Can you work these out from the model? Positions are in its coordinate system, mm. A direction names the side the tool comes from. Give positions to 0.01 mm unless a question says otherwise; leave off trailing zeros. Loops run counter-clockwise (first coordinate to the right, second up) from the corner with the lowest first, then second, coordinate; pieces in that order, holes last.
from build123d import *

# Parameters (mm, degrees)
SKETCH_1_R           = 6
EXTRUDE_1_DEPTH      = 2
SKETCH_2_R           = 3.5
EXTRUDE_2_DEPTH      = 12.5
EXTRUDE_START        = -2.5
EXTRUDE_3_DEPTH      = 2.5
EXTRUDE_4_DEPTH      = 0.5
EXTRUDE_4_DEPTH_BACK = 0.5
SKETCH_5_R           = 3
EXTRUDE_5_DEPTH      = 0.5
SKETCH_6_R           = 2
EXTRUDE_6_DEPTH      = 16
SKETCH_8_W           = 1
SKETCH_8_H           = 6
CUT_EXTRUDE_1_DEPTH  = 6
CUT_EXTRUDE_2_DEPTH  = 24.092206478
FILLET_1_R           = 0.2
CHAMFER_1_SIZE       = 0.5


with BuildPart() as part:
    # 草图1 → 凸台-拉伸1 (new body)
    with BuildSketch(Plane(origin=(0, 0, 0), x_dir=(1, 0, 0), z_dir=(0, 1, 0))):
        with Locations(Location((0, 0, 0), (0, 0, 270))):
            Circle(SKETCH_1_R)
    extrude(amount=EXTRUDE_1_DEPTH)

    # 草图2 → 凸台-拉伸2 (add)
    with BuildSketch(Plane(origin=(0, 2, 0), x_dir=(1, 0, 0), z_dir=(0, 1, 0))):
        with Locations(Location((0, 0, 0), (0, 0, 270))):
            Circle(SKETCH_2_R)
    extrude(amount=EXTRUDE_2_DEPTH)

    # 草图3 → 凸台-拉伸3 (add)
    with BuildSketch(Plane(origin=(0, 14.5, 0), x_dir=(1, 0, 0), z_dir=(0, 1, 0)).offset(EXTRUDE_START)):
        with BuildLine():
            Line((-12.125, 2.997394702), (-0.145833333, 3.496960486))
            ThreePointArc((-0.145833333, 3.496960486), (3.5, 0), (-0.145833333, -3.496960486))
            Line((-0.145833333, -3.496960486), (-12.125, -2.997394702))
            ThreePointArc((-12.125, -2.997394702), (-15, 0), (-12.125, 2.997394702))
        make_face()
    extrude(amount=EXTRUDE_3_DEPTH)

    # 草图4 → 凸台-拉伸4 (add, two sides: drawn at the far end of the back side and taken through both)
    with BuildSketch(Plane.XY.offset(-EXTRUDE_4_DEPTH_BACK)):
        Polygon((-14.2, 12), (-3.2, 8), (-0.2, 6.909090909), (-0.2, 12), (-3.2, 12), align=None)
    extrude(amount=EXTRUDE_4_DEPTH + EXTRUDE_4_DEPTH_BACK)

    # 草图5 → 凸台-拉伸5 (add)
    with BuildSketch(Plane(origin=(0, 14.5, 0), x_dir=(1, 0, 0), z_dir=(0, 1, 0))):
        with Locations(Location((-12, 0, 0), (0, 0, 270))):
            Circle(SKETCH_5_R)
    extrude(amount=EXTRUDE_5_DEPTH)

    # 草图6 → 凸台-拉伸6 (add)
    with BuildSketch(Plane(origin=(0, 15, 0), x_dir=(1, 0, 0), z_dir=(0, 1, 0))):
        with Locations(Location((-12, 0, 0), (0, 0, 270))):
            Circle(SKETCH_6_R)
    extrude(amount=EXTRUDE_6_DEPTH)

    # 草图7 → 旋转1 (revolve)
    with BuildSketch(Plane.XY, mode=Mode.PRIVATE) as revolve_1_sk:
        Polygon((-12, 31), (-14, 31), (-14.1, 30), (-12, 30), align=None)
    revolve(revolve_1_sk.sketch.rotate(Axis((-12, 30, 0), (0, 1, 0)), 90), axis=Axis((-12, 30, 0), (0, 1, 0)))

    # 草图8 → 切除-拉伸1 (cut)
    with BuildSketch(Plane(origin=(0, 31, 0), x_dir=(1, 0, 0), z_dir=(0, 1, 0))):
        with Locations((-12, 0)):
            Rectangle(SKETCH_8_W, SKETCH_8_H)
    extrude(amount=-CUT_EXTRUDE_1_DEPTH, mode=Mode.SUBTRACT)

    # 草图9 → 切除-拉伸2 (cut, through all)
    with BuildSketch(Plane(origin=(0, 14.5, 0), x_dir=(1, 0, 0), z_dir=(0, 1, 0))):
        with BuildLine():
            Line((1.519868415, -1.3), (-1.519868415, -1.3))
            ThreePointArc((-1.519868415, -1.3), (-2, 0), (-1.519868415, 1.3))
            Line((-1.519868415, 1.3), (1.519868415, 1.3))
            ThreePointArc((1.519868415, 1.3), (2, 0), (1.519868415, -1.3))
        make_face()
    extrude(amount=-CUT_EXTRUDE_2_DEPTH, mode=Mode.SUBTRACT)

    # 圆角1
    fillet_1_edges = [part.edges().sort_by_distance(p)[0] for p in [
        (0, 0, -6),
        (0, 2, -6),
    ]]
    fillet(fillet_1_edges, radius=FILLET_1_R)

    # 倒角1
    # the kernel refuses this chamfer: 0.5 mm, written as the material it takes off along each edge
    with BuildSketch(Plane(origin=(1.138891494, 12, 3.550537215), x_dir=(-0.0011456615254410918, 0.9996219169112968, 0.02747199829378469), z_dir=(-0.9991315673568166, 0, -0.041666666666666574))) as chamfer_1_piece_1_section:
        Polygon((CHAMFER_1_SIZE * 0.999621916911, CHAMFER_1_SIZE * 0.0274958766106), (-CHAMFER_1_SIZE * 0.0274958766106, CHAMFER_1_SIZE * 0.999621916911), (0, 0), align=None)
    chamfer_1_piece_1 = extrude(amount=13.275420302, mode=Mode.PRIVATE)
    chamfer_1_piece_1 = chamfer_1_piece_1 - Plane(origin=(0, 12.171019003, 0), x_dir=(0, 0, 1), z_dir=(0, -1, 0)) * Cylinder(3.5, 29, mode=Mode.PRIVATE)
    add(chamfer_1_piece_1, mode=Mode.SUBTRACT)
    with BuildSketch(Plane(origin=(-12, 12, 0), x_dir=(-0.041666666666666664, 0, 0.9991315673568165), z_dir=(0.9991315673568165, 0, 0.041666666666666664))) as chamfer_1_piece_2:
        Polygon((3 - CHAMFER_1_SIZE, 0), (3, -CHAMFER_1_SIZE), (3, 0), align=None)
    revolve(axis=Axis((-12, 12, 0), (0, -1, 0)), revolution_arc=175.223969073, mode=Mode.SUBTRACT)
    with BuildSketch(Plane(origin=(-12.125, 12, -2.997394702), x_dir=(0.04165091320463745, -0.027495876610585623, 0.9987538126078094), z_dir=(0.9991315673568165, 0, -0.041666666666666755))) as chamfer_1_piece_3_section:
        Polygon((CHAMFER_1_SIZE * 0.999621916911, -CHAMFER_1_SIZE * 0.0274958766106), (-CHAMFER_1_SIZE * 0.0274958766106, -CHAMFER_1_SIZE * 0.999621916911), (0, 0), align=None)
    chamfer_1_piece_3 = extrude(amount=13.275420302, mode=Mode.PRIVATE)
    chamfer_1_piece_3 = chamfer_1_piece_3 - Plane(origin=(0, 12.143445787, 0), x_dir=(0, 0, 1), z_dir=(0, -1, 0)) * Cylinder(3.5, 29, mode=Mode.PRIVATE)
    add(chamfer_1_piece_3, mode=Mode.SUBTRACT)
    with BuildSketch(Plane(origin=(-13.409724827, 14.5, -2.943817973), x_dir=(0.04165091320463745, 0.027495876610585623, 0.9987538126078094), z_dir=(0.9991315673568165, 0, -0.041666666666666755))) as chamfer_1_piece_4_section:
        Polygon((CHAMFER_1_SIZE * 0.999621916911, CHAMFER_1_SIZE * 0.0274958766106), (-CHAMFER_1_SIZE * 0.0274958766106, CHAMFER_1_SIZE * 0.999621916911), (0, 0), align=None)
    chamfer_1_piece_4 = extrude(amount=13.275420302, mode=Mode.PRIVATE)
    chamfer_1_piece_4 = chamfer_1_piece_4 - Plane(origin=(-12, 14.328980995, 0), x_dir=(0, 0, 1), z_dir=(0, -1, 0)) * Cylinder(3, 29, mode=Mode.PRIVATE)
    add(chamfer_1_piece_4, mode=Mode.SUBTRACT)
    with BuildSketch(Plane(origin=(0, 14.5, 0), x_dir=(0, 0, 1), z_dir=(-1, 0, 0))) as chamfer_1_piece_5:
        Polygon((3.5, -CHAMFER_1_SIZE), (3.5 - CHAMFER_1_SIZE, 0), (3.5, 0), align=None)
    revolve(axis=Axis((0, 14.5, 0), (0, 1, 0)), revolution_arc=182.388015463, mode=Mode.SUBTRACT)
    with BuildSketch(Plane(origin=(-0.145833333, 14.5, 3.496960486), x_dir=(0.04165091320463727, 0.027495876610585623, -0.9987538126078094), z_dir=(-0.9991315673568166, 0, -0.041666666666666574))) as chamfer_1_piece_6_section:
        Polygon((CHAMFER_1_SIZE * 0.999621916911, CHAMFER_1_SIZE * 0.0274958766106), (-CHAMFER_1_SIZE * 0.0274958766106, CHAMFER_1_SIZE * 0.999621916911), (0, 0), align=None)
    chamfer_1_piece_6 = extrude(amount=13.275420302, mode=Mode.PRIVATE)
    chamfer_1_piece_6 = chamfer_1_piece_6 - Plane(origin=(-12, 14.356641066, 0), x_dir=(0, 0, 1), z_dir=(0, -1, 0)) * Cylinder(3, 29, mode=Mode.PRIVATE)
    add(chamfer_1_piece_6, mode=Mode.SUBTRACT)
    with BuildSketch(Plane(origin=(0, 14.5, 0), x_dir=(-0.04166666666666704, 0, 0.9991315673568166), z_dir=(-0.9991315673568166, 0, -0.04166666666666704))) as chamfer_1_piece_7:
        Polygon((3.5, -CHAMFER_1_SIZE), (3.5 - CHAMFER_1_SIZE, 0), (3.5, 0), align=None)
    revolve(axis=Axis((0, 14.5, 0), (0, 1, 0)), revolution_arc=2.388015463, mode=Mode.SUBTRACT)


solid = part.part
(1) Thinking about a two-plate mould opening in X: for faces 5 (the cylindrical face through (1.802, 0.989, 5.723)), 6 (the flat face through (-12.5, 28, 0)), 7 (the flat face through (-13, 31, 0)), which applies, pulls with the +X half, pulls with the -X half, needs draft (parallel to the pull), parting line crosses it, or undercut?
Returned:
face 5: parting line crosses it
face 6: undercut
face 7: needs draft
(2) Suppose I cut it at A-A on y = 5.5. List the corners of the cut face in (x, z) for me, plus the area to 3 significant figures.
Returned:
outline: circle Ø7 at (0, 0); hole (-1.52, -1.3) - (1.52, -1.3) arc R2 ccw to (1.52, 1.3) - (-1.52, 1.3) arc R2 ccw to start
area: 28.9 mm2
(3) Suppose I cut it at B-B on y = 29. List the corners of the cut face in (x, z) for me, plus the area to 3 significant figures.
Returned:
outline: (-12.5, -1.94) - (-12.5, 1.94) arc R2 ccw to start; (-11.5, -1.94) arc R2 ccw to (-11.5, 1.94) - close
area: 8.61 mm2
(4) Suppose I cut it at C-C on y = 18. List the corners of the cut face in (x, z) for me.
Returned:
outline: circle Ø4 at (-12, 0)
(5) Which directions (+Z, -Z, +X, -X, +Y, -Y) give clear straight access to the entire face, cutting with the end or side of a thin tool? Please do faces 1 (the flat face through (-7, 11, 0.5)), 2 (the flat face through (-6.05, 13.24, 3.25)), 3 (the flat face through (-6.219, 13.239, -3.244)), 4 (the flat face through (-12, 25, 0)).
Returned:
face 1: +Z, -X
face 2: +Z, -X, +Y
face 3: -Z, -X, +Y
face 4: +Z, -Z, +Y
(6) Will these pins go through, and if not, where does the flat tip stop? P1, Ø1.5, axis at x = -4, z = -0.5, coming from the +Y side; P2, Ø4.5, axis at x = -8.5, y = 10, coming from the +Z side; P3, Ø2, axis at x = -5.5, y = 13, coming from the -Z side.
Returned:
P1: stops at y = 14.5
P2: stops at z = 2.9
P3: stops at z = -3.32
(7) Please list where these lines run through material, in increasing order: probe 1 along Y at (x, z) = (-5.25, 2.5); probe 2 along Y at (x, z) = (3.75, 3.75); probe 3 along X at (y, z) = (6, 1).
Returned:
probe 1: y = 0 to 2, 12 to 14.5
probe 2: y = 0 to 2
probe 3: x = -3.35 to -1.73, 1.73 to 3.35
